Part model, mm, in its own coordinate system. A direction names the side the tool comes from. Round coordinates to 2 decimals unless told otherwise and drop trailing zeros. Write each loop counter-clockwise with the first axis right and the second up, starting at its lowest first coordinate (ties: lowest second). Pieces come first, ordered by that corner, then holes.
```python
from build123d import *

# Parameters (mm, degrees)
SKETCH1_R            = 60
BOSS_EXTRUDE1_DEPTH  = 2
SKETCH4_R            = 40.5
SKETCH4_R_2          = 37.5
BOSS_EXTRUDE4_DEPTH  = 0.3
SKETCH5_R            = 1.75
BOSS_EXTRUDE5_DEPTH  = 0.3
CIRPATTERN1_COUNT    = 4
SKETCH6_R            = 1.75
CUT_EXTRUDE1_DEPTH   = 85.876380696
BOSS_EXTRUDE6_DEPTH  = 5
SKETCH8_R            = 1.337594407
CUT_EXTRUDE2_DEPTH   = 109.252020766
FILLET1_R            = 5
FILLET1_OF_MIRROR1_R = 5


with BuildPart() as part:
    # Sketch1 → Boss-Extrude1 (new body)
    with BuildSketch(Plane.XY):
        Circle(SKETCH1_R)
    extrude(amount=BOSS_EXTRUDE1_DEPTH)

    # Sketch4 → Boss-Extrude4 (add)
    with BuildSketch(Plane.XY.offset(2)):
        Circle(SKETCH4_R)
        Circle(SKETCH4_R_2, mode=Mode.SUBTRACT)
    extrude(amount=BOSS_EXTRUDE4_DEPTH)

    # Sketch5 → Boss-Extrude5 (add)
    with BuildSketch(Plane.XY.offset(2)):
        with BuildLine():
            Line((-7.5, 39.799497484), (7.5, 39.799497484))
            Line((7.5, 39.799497484), (3.715004122, 49.282313849))
            ThreePointArc((3.715004122, 49.282313849), (0, 51.799497484), (-3.715004122, 49.282313849))
            Line((-3.715004122, 49.282313849), (-7.5, 39.799497484))
        make_face()
        with Locations((0, 47.799497484)):
            Circle(SKETCH5_R, mode=Mode.SUBTRACT)
    boss_extrude5 = extrude(amount=BOSS_EXTRUDE5_DEPTH)

    # CirPattern1: Boss-Extrude5 ×4 about axis
    cirpattern1_axis = Axis((0, 0, 0), (0, 0, 1))
    for i in range(1, CIRPATTERN1_COUNT):
        add(boss_extrude5.rotate(cirpattern1_axis, i * 360 / CIRPATTERN1_COUNT))

    # Sketch6 → Cut-Extrude1 (cut, through all)
    with BuildSketch(Plane.XY.offset(2)):
        with Locations((0, 47.799497484)):
            Circle(SKETCH6_R)
        with Locations(Location((-47.799497484, 0, 0), (0, 0, 90))):
            Circle(SKETCH6_R)
        with Locations(Location((47.799497484, 0, 0), (0, 0, 270))):
            Circle(SKETCH6_R)
        with Locations(Location((0, -47.799497484, 0), (0, 0, 180))):
            Circle(SKETCH6_R)
    extrude(amount=-CUT_EXTRUDE1_DEPTH, mode=Mode.SUBTRACT)

    # Sketch7 → Boss-Extrude6 (add, symmetric)
    with BuildSketch(Plane(origin=(0, 0, 0), x_dir=(1, 0, 0), z_dir=(0, 1, 0))):
        Polygon((60, 0), (81.5, -21.5), (87.5, -21.5), (87.5, -24.5), (77.428932188, -24.5), (52.928932188, 0), align=None)
    boss_extrude6 = extrude(amount=BOSS_EXTRUDE6_DEPTH, both=True)

    # Sketch8 → Cut-Extrude2 (cut, through all)
    with BuildSketch(Plane(origin=(0, 0, 21.5), x_dir=(-1, 0, 0), z_dir=(0, 0, -1))):
        with Locations((-84.5, 0)):
            Circle(SKETCH8_R)
    cut_extrude2 = extrude(amount=-CUT_EXTRUDE2_DEPTH, mode=Mode.SUBTRACT)

    # Fillet1
    fillet1_edges = [part.edges().sort_by_distance(p)[0] for p in [
        (87.5, -5, 23),
        (87.5, 5, 23),
    ]]
    fillet(fillet1_edges, radius=FILLET1_R - 0.0001)  # a hair under: the kernel refuses the full size

    # Mirror1: Boss-Extrude6, Cut-Extrude2 across plane
    add(boss_extrude6.mirror(Plane(origin=(0, 0, 0), x_dir=(0, 0, 1), z_dir=(1, 0, 0))))
    add(cut_extrude2.mirror(Plane(origin=(0, 0, 0), x_dir=(0, 0, 1), z_dir=(1, 0, 0))), mode=Mode.SUBTRACT)

    # Fillet1 of Mirror1
    fillet1_of_mirror1_edges = [part.edges().sort_by_distance(p)[0] for p in [
        (-87.5, -5, 23),
        (-87.5, 5, 23),
    ]]
    fillet(fillet1_of_mirror1_edges, radius=FILLET1_OF_MIRROR1_R - 0.0001)  # a hair under: the kernel refuses the full size


solid = part.part
```
Q1. Cut at B-B on z = 5. Write the cut outline in (x, y).
Values follow:
outline: (-65, -5) - (-57.93, -5) - (-57.93, 5) - (-65, 5) - close; (57.93, -5) - (65, -5) - (65, 5) - (57.93, 5) - close
Q2. Drop flat-ended pins along their axis: pin 1 (12 mm diameter, centred on x = 21.5, z = 5, fed in from -Y); pin 2 (1 mm diameter, centred on x = -30, y = 17, fed in from +Z); pin 3 (2 mm diameter, centred on x = 0, y = -47.8, fed in from +Z); pin 4 (3 mm diameter, centred on x = 83.5, y = -2, fed in from -Z). Give the stop position or say it passes through.
Values follow:
pin 1: stops at y = -57.74
pin 2: stops at z = 2
pin 3: passes through
pin 4: stops at z = 21.5
Q3. Cut at D-D on x = -18.5. Write the cut outline in (y, z).
Values follow:
outline: (-57.08, 0) - (57.08, 0) - (57.08, 2) - (36.03, 2) - (36.03, 2.3) - (32.62, 2.3) - (32.62, 2) - (-32.62, 2) - (-32.62, 2.3) - (-36.03, 2.3) - (-36.03, 2) - (-57.08, 2) - close
Q4. Wall check: L1, parallel to Y at x = 0, z = 2.2; L2, parallel to Z at x = -39, y = 0.5; L3, parallel to Z at x = -49, y = 23.5. Give the ranges that are in metal, low to high.
Values follow:
L1: y = -51.8 to -49.55, -46.05 to -37.5, 37.5 to 46.05, 49.55 to 51.8
L2: z = 0 to 2.3
L3: z = 0 to 2
Q5. Mould opens along X. For faces 1 (the flat face through (-71, 0, 11)), 2 (the flat face through (-83, 0, 21.5)), 3 (the flat face through (27, -27, 2.3)), 4 (the flat face through (-66.34, 0.07, 13.41)) say: +X half, -X half, draft (parallel to the pull), parting line (faces both ways), or undercut.
Values follow:
face 1: -X half
face 2: draft
face 3: undercut
face 4: undercut
Q6. Cut at C-C on y = 32. Write the cut outline in (x, z), plus the area to 3 significant figures.
Values follow:
outline: (-50.75, 0) - (50.75, 0) - (50.75, 2) - (24.82, 2) - (24.82, 2.3) - (19.55, 2.3) - (19.55, 2) - (-19.55, 2) - (-19.55, 2.3) - (-24.82, 2.3) - (-24.82, 2) - (-50.75, 2) - close
area: 206 mm2
Q7. Which spindle directions (+Z, -Z, +X, -X, +Y, -Y) get a long thin tool onto all of the face, cutting with end or side? Do faces 5 (the flat face through (66.34, 0.07, 13.41)), 6 (the cylindrical face through (-86, 3.57, 23.02)). Say none if no direction does.
Values follow:
face 5: +Z, +Y, -Y
face 6: +Z, -Z, -X, +Y
Q8. Cut at A-A on x = 0. Write the cut outline in (y, z), plus the area to 3 significant figures.
Values follow:
outline: (-60, 0) - (-49.55, 0) - (-49.55, 2.3) - (-51.8, 2.3) - (-51.8, 2) - (-60, 2) - close; (-46.05, 0) - (46.05, 0) - (46.05, 2.3) - (37.5, 2.3) - (37.5, 2) - (-37.5, 2) - (-37.5, 2.3) - (-46.05, 2.3) - close; (49.55, 0) - (60, 0) - (60, 2) - (51.8, 2) - (51.8, 2.3) - (49.55, 2.3) - close
area: 232 mm2
